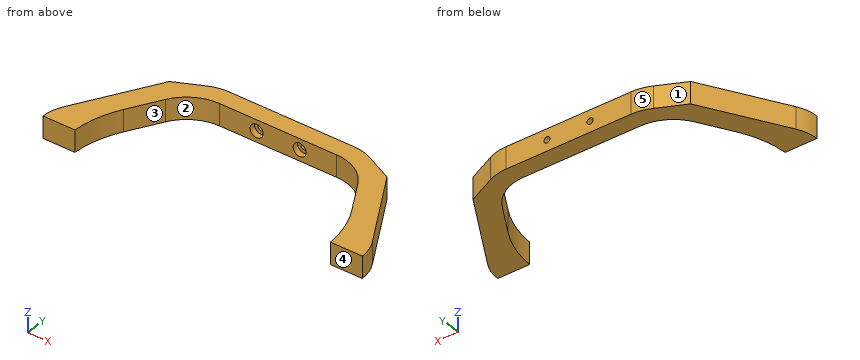
```python
from build123d import *

# Parameters (mm, degrees)
BOSS_EXTRUDE1_DEPTH = 7.5
CUT_EXTRUDE1_START  = 80.121778
SKETCH3_R           = 2.1
CUT_EXTRUDE1_DEPTH  = 12
FILLET1_R           = 30
FILLET1_R_2         = 70
FILLET2_R           = 30
FILLET2_R_2         = 28
CUT_EXTRUDE2_START  = 72.121778
SKETCH3_4_R         = 4.5
SKETCH3_4_R_2       = 2.1
CUT_EXTRUDE2_DEPTH  = 6


with BuildPart() as part:
    # Sketch2 → Boss-Extrude1 (new, symmetric)
    with BuildSketch(Plane.XY):
        Polygon((-50, 80.121778265), (-75, 68.121778265), (-110, 7.5), (-110, 0), (-88.009618943, 0), (-88.009618943, 15.588457268), (-57.679491924, 68.121778265), (57.679491924, 68.121778265), (88.009618943, 15.588457268), (88.009618943, 0), (110, 0), (110, 7.5), (75, 68.121778265), (50, 80.121778265), align=None)
    extrude(amount=BOSS_EXTRUDE1_DEPTH, both=True)

    # Sketch3 → Cut-Extrude1 (cut)
    with BuildSketch(Plane(origin=(0, 0, 0), x_dir=(1, 0, 0), z_dir=(0, 1, 0)).offset(CUT_EXTRUDE1_START)):
        with Locations(Location((-14.832079928, 0, 0), (0, 0, 270))):
            Circle(SKETCH3_R)
        with Locations(Location((14.832079928, 0, 0), (0, 0, 270))):
            Circle(SKETCH3_R)
    extrude(amount=-CUT_EXTRUDE1_DEPTH, mode=Mode.SUBTRACT)

    # Fillet1
    # the kernel refuses this fillet: 70, 30 mm, written as the material it adds along each edge
    with BuildSketch(Plane(origin=(-57.679491924, 68.121778265, -7.5), x_dir=(-0.500000000000001, -0.8660254037844382, 0), z_dir=(0, 0, 1)), Plane(origin=(57.679491924, 68.121778265, -7.5), x_dir=(-1, 0, 0), z_dir=(0, 0, 1))) as fillet1_piece_1:
        with BuildLine():
            CenterArc((FILLET1_R * 0.57735026919, FILLET1_R), FILLET1_R, 210, 60)
            Line((-FILLET1_R * 0.288675134595, FILLET1_R * 0.5), (-FILLET1_R * 0.305995642671, FILLET1_R * 0.49))
            Line((-FILLET1_R * 0.305995642671, FILLET1_R * 0.49), (-FILLET1_R * 0.0115470053838, -FILLET1_R * 0.02))
            Line((-FILLET1_R * 0.0115470053838, -FILLET1_R * 0.02), (FILLET1_R * 0.57735026919, -FILLET1_R * 0.02))
            Line((FILLET1_R * 0.57735026919, -FILLET1_R * 0.02), (FILLET1_R * 0.57735026919, 0))
        make_face()
    extrude(amount=15)
    with BuildSketch(Plane(origin=(-88.009618943, 15.588457268, -7.5), x_dir=(0, -1, 0), z_dir=(0, 0, 1))) as fillet1_piece_2:
        with BuildLine():
            CenterArc((18.891495711, 69.922027552), FILLET1_R_2, 240, 27.295421975)
            Line((-16.108504289, 9.300249288), (-16.808504289, 8.087813722))
            Line((-16.808504289, 8.087813722), (-0.7, -1.212435565))
            Line((-0.7, -1.212435565), (0, -1.4))
            ThreePointArc((0, -1.4), (7.794228634, -1.4), (15.522396499, -1.398440551))
            Line((15.522396499, -1.398440551), (15.588457268, 0))
        make_face()
    extrude(amount=15)
    with BuildSketch(Plane(origin=(88.009618943, 15.588457268, 7.5), x_dir=(-0.5000000000000018, 0.8660254037844377, 0), z_dir=(0, 0, -1))) as fillet1_piece_3:
        with BuildLine():
            CenterArc((18.600498575, -70), FILLET1_R_2, 90, 27.295421975)
            Line((-13.5, -7.794228634), (-14.142009972, -6.550113207))
            ThreePointArc((-14.142009972, -6.550113207), (-7.45, -2.684678752), (-0.7, 1.212435565))
            Line((-0.7, 1.212435565), (0, 1.4))
            Line((0, 1.4), (18.600498575, 1.4))
            Line((18.600498575, 1.4), (18.600498575, 0))
        make_face()
    extrude(amount=15)

    # Fillet2
    # the kernel refuses this fillet: 30, 28 mm, written as the material it takes off along each edge
    with BuildSketch(Plane(origin=(-50, 80.121778265, -24.567807798), x_dir=(1, 0, 0), z_dir=(0, 0, 1)), Plane(origin=(50, 80.121778265, -24.567807798), x_dir=(0.9015230574682733, -0.43273106758477164, 0), z_dir=(0, 0, 1))) as fillet2_piece_1:
        with BuildLine():
            CenterArc((FILLET2_R * 0.227570770644, -FILLET2_R), FILLET2_R, 90, 25.641005824)
            Line((-FILLET2_R * 0.205160296941, -FILLET2_R * 0.0984769425317), (0, 0))
            Line((0, 0), (FILLET2_R * 0.227570770644, 0))
        make_face()
    extrude(amount=49.135615597, mode=Mode.SUBTRACT)
    with BuildSketch(Plane(origin=(-110, 7.5, -26.25644347), x_dir=(0.5000000000000017, 0.8660254037844376, 0), z_dir=(0, 0, 1)), Plane(origin=(110, 7.5, -26.25644347), x_dir=(0, -1, 0), z_dir=(0, 0, 1))) as fillet2_piece_2:
        with BuildLine():
            CenterArc((FILLET2_R_2 * 0.267949192431, -FILLET2_R_2), FILLET2_R_2, 90, 30)
            Line((-FILLET2_R_2 * 0.232050807569, -FILLET2_R_2 * 0.133974596216), (0, 0))
            Line((0, 0), (FILLET2_R_2 * 0.267949192431, 0))
        make_face()
    extrude(amount=52.51288694, mode=Mode.SUBTRACT)

    # Sketch3<4> → Cut-Extrude2 (cut)
    # profile 1 of 2: a face of its own
    with BuildSketch(Plane(origin=(0, 0, 0), x_dir=(1, 0, 0), z_dir=(0, 1, 0)).offset(CUT_EXTRUDE2_START)):
        with Locations(Location((-14.832079928, 0, 0), (0, 0, 90))):
            Circle(SKETCH3_4_R)
        with Locations(Location((-14.832079928, 0, 0), (0, 0, 270))):
            Circle(SKETCH3_4_R_2, mode=Mode.SUBTRACT)
    # profile 2 of 2: a face of its own
    with BuildSketch(Plane(origin=(0, 0, 0), x_dir=(1, 0, 0), z_dir=(0, 1, 0)).offset(CUT_EXTRUDE2_START)):
        with Locations(Location((14.832079928, 0, 0), (0, 0, 90))):
            Circle(SKETCH3_4_R)
        with Locations(Location((14.832079928, 0, 0), (0, 0, 270))):
            Circle(SKETCH3_4_R_2, mode=Mode.SUBTRACT)
    extrude(amount=-CUT_EXTRUDE2_DEPTH, mode=Mode.SUBTRACT)


solid = part.part
```
Geometry check sheet. Reference: the model listing, model coordinates, mm. Face numbers are marked on the shaded views. A direction names the side the tool comes from. Coordinates: 2 decimals unless noted, no trailing zeros. Loops run counter-clockwise (first coordinate to the right, second up) from the corner with the lowest first, then second, coordinate; pieces in that order, holes last. Notation, with made-up numbers: (-29, 11) - (14, 11) arc R14 ccw to (14, 19) - close; hole circle Ø11 at (-37, 34.5). An arc over 180 degrees is marked (long way). One line per item, written item: value. Start each with the question number.
(1) Cross-section at B-B on y = 43. Enter the section's corners in (x, z).
(2) Cross-section at D-D on x = -93.5. Enter the section's corners in (y, z), plus the area to 3 significant figures.
(3) Depth check by flat-ended pin: P1, Ø7, axis at x = 17, z = -2, coming from the -Y side; P2, Ø6, axis at y = 12.5, z = 2.5, coming from the +X side; P3, Ø6, axis at y = 62.5, z = 4, coming from the +X side. Enter the tip coordinate at first touch or a pass-through.
(4) Material ranges on line 1 (X direction, y = 75, z = 0); line 2 (X direction, y = 70, z = -2); line 3 (X direction, y = 35.5, z = -5.75), recorded low to high. Write a range as [from, to].
(5) Mould release check, pull along X, two halves, no side actions. Record for the marked faces 3, 4 and 5: released by +X, released by -X, zero draft, split by the parting line, or undercut.
(6) Tool access check on the marked faces 1 and 2. Record the directions out of +Z, -Z, +X, -X, +Y, -Y that give a thin tool (end or side, any length) a straight path to the whole face; none if there is none.
(7) Cross-section at A-A on z = 0. Count the separate pieces of the cut face and the enclosed holes in it, plus the area to 3 significant figures.
(8) Cross-section at C-C on x = -4. Enter the section's corners in (y, z).
Results below:
1. outline: (-89.5, -7.5) - (-72.18, -7.5) - (-72.18, 7.5) - (-89.5, 7.5) - close; (72.18, -7.5) - (89.5, -7.5) - (89.5, 7.5) - (72.18, 7.5) - close
2. outline: (0, -7.5) - (36.08, -7.5) - (36.08, 7.5) - (0, 7.5) - close
2. area: 541 mm2
3. P1: stops at y = 68.12
3. P2: stops at x = 108.34
3. P3: stops at x = 79.98
4. line 1: x = [-60.67, -16.93], [-12.73, 12.73], [16.93, 60.67]
4. line 2: x = [-71.09, -18.86], [-10.8, 10.8], [18.86, 71.09]
4. line 3: x = [-93.83, -76.51], [76.51, 93.83]
5. face 3: undercut
5. face 4: zero draft
5. face 5: released by -X
6. face 1: +Z, -Z, -X, +Y
6. face 2: +Z, -Z, -Y
7. separate pieces: 3
7. enclosed holes: 0
7. area: 3,970 mm2
8. outline: (68.12, -7.5) - (80.12, -7.5) - (80.12, 7.5) - (68.12, 7.5) - close
